Autodesk Inventor part; units mm, degrees
ref_plane "YZ Plane" through (0, 0, 0) normal (1, 0, 0) x (0, 1, 0)
ref_plane "XZ Plane" through (0, 0, 0) normal (0, 1, 0) x (-1, 0, 0)
ref_plane "XY Plane" through (0, 0, 0) normal (0, 0, 1) x (1, 0, 0)
sketch "スケッチ2" plane through (0, 0, 0) normal (0, 1, 0) x (-1, 0, 0)
  line L0 (0, 0) -> (20.1, 0)
  line L1 (20.1, 0) -> (20.1, -40)
  line L2 (20.1, -40) -> (0, -40)
  line L3 (0, -40) -> (0, 0)
  dimension "d0" = 20.1
  dimension "d1" = 40
extrude "押し出し1" add sketch "スケッチ2" along normal blind 27.5
ref_plane "作業平面1" through (0, 27.5, 0) normal (0, 1, 0) x (1, 0, 0)
sketch "スケッチ3" plane through (0, 27.5, 0) normal (0, 1, 0) x (1, 0, 0)
  line L0 (-20.1, 47.19) -> (0, 47.19)
  line L1 (0, 47.19) -> (0, -7.19)
  line L2 (0, -7.19) -> (-20.1, -7.19)
  line L3 (-20.1, -7.19) -> (-20.1, 47.19)
  line L4 (-20.1, 40) -> (-20.1, 0)
  line L5 (0, 40) -> (-20.1, 40)
  point P0 (0, 0)
  point P1 (-20.1, 20)
  point P2 (-20.1, 20)
  point P3 (-10.05, 47.19)
  point P4 (-10.05, 40)
  point P5 (-10.05, 40)
  point P6 (0, 40)
  point P7 (-20.1, 40)
  dimension "d5" = 20.1
  dimension "d6" = 54.38
  dimension "d7" = 0
  dimension "d8" = 0
extrude "押し出し2" add sketch "スケッチ3" along normal blind 3.1
ref_plane "作業平面2" through (0, 30.6, 0) normal (0, 1, 0) x (1, 0, 0)
sketch "スケッチ4" plane through (0, 30.6, 0) normal (0, 1, 0) x (1, 0, 0)
  line L0 (0, -7.19) -> (0, 0)
  line L1 (0, 0) -> (-20.1, 0)
  line L2 (-20.1, 0) -> (-20.1, 40)
  line L3 (-20.1, 40) -> (0, 40)
  line L4 (0, 40) -> (0, 0)
  circle A0 centre (-14.9, 45.43) radius 2
  circle A1 centre (-5.2, 45.43) radius 2
  line L5 (-15.85, 47.19) -> (-13.95, 47.19)
  line L6 (-6.15, 47.19) -> (-4.25, 47.19)
  line L7 (-13.95, 47.19) -> (-6.15, 47.19)
  line L8 (0, 47.19) -> (-20.1, 47.19)
  point P0 (-10.05, 47.19)
  dimension "d12" = 40
  dimension "d23" = 4
  dimension "d24" = 4
  dimension "d27" = 1.9
  dimension "d28" = 1.9
  dimension "d29" = 7.8
  dimension "d53" = 20.1
extrude "押し出し3" add sketch "スケッチ4" along normal blind 9.55 contours L1 L2 L3 L4
sketch "スケッチ7" plane through (0, 30.6, 0) normal (0, 1, 0) x (1, 0, 0)
  circle A0 centre (-14.9, 45.43) radius 2
  circle A1 centre (-5.2, 45.43) radius 2
  circle A2 centre (-14.9, -5.43) radius 2
  circle A3 centre (-5.2, -5.43) radius 2
  line L0 (-13.95, 47.19) -> (-15.85, 47.19)
  line L1 (-6.15, 47.19) -> (-4.25, 47.19)
  line L2 (-15.85, -7.19) -> (-13.95, -7.19)
  line L3 (-6.15, -7.19) -> (-4.25, -7.19)
  line L4 (-13.95, -7.19) -> (-6.15, -7.19)
  line L5 (-13.95, 47.19) -> (-6.15, 47.19)
  line L6 (0, 47.19) -> (-20.1, 47.19)
  line L7 (-20.1, -7.19) -> (0, -7.19)
  point P0 (0, 0)
  point P1 (-10.05, -7.19)
  point P2 (-10.05, 47.19)
  point P3 (-10.05, -7.19)
  dimension "d33" = 4
  dimension "d34" = 4
  dimension "d35" = 4
  dimension "d36" = 4
  dimension "d37" = 1.9
  dimension "d38" = 1.9
  dimension "d39" = 1.9
  dimension "d40" = 1.9
  dimension "d41" = 7.8
  dimension "d42" = 7.8
extrude "押し出し6" cut sketch "スケッチ7" against normal through all contours A0 L0 | L1 A1 | A2 L2 | A3 L3 | L3 A3 | L2 A2 picked at (-15.3262, 45.9006) picked at (-5.6145, 46.6348)
ref_plane "作業平面5" through (-20.1, 0, 0) normal (0, 0, 1) x (1, 0, 0)
sketch "スケッチ8" plane through (-20.1, 0, 0) normal (0, 0, 1) x (1, 0, 0)
  line L0 (6.05, 11.2) -> (14.05, 11.2)
  line L1 (14.05, 11.2) -> (14.05, 6.5)
  line L2 (14.05, 6.5) -> (6.05, 6.5)
  line L3 (6.05, 6.5) -> (6.05, 11.2)
  line L4 (0, 0) -> (0, 27.5)
  line L5 (20.1, 0) -> (20.1, 27.5)
  line L6 (0, 0) -> (20.1, 0)
  dimension "d46" = 8
  dimension "d47" = 4.7
  dimension "d48" = 6.05
  dimension "d49" = 6.05
  dimension "d50" = 6.5
extrude "押し出し7" cut sketch "スケッチ8" against normal blind 4.15
ref_plane "作業平面6" through (0, 40.15, 0) normal (0, 1, 0) x (1, 0, 0)
sketch "スケッチ10" plane through (0, 40.15, 0) normal (0, 1, 0) x (1, 0, 0)
  line L0 (-20.1, 0) -> (0, 0)
  circle A0 centre (-10.05, 9.9) radius 2.5
  point P0 (-10.05, 0)
  dimension "d57" = 9.9
  dimension "d59" = 5
extrude "押し出し8" add sketch "スケッチ10" along normal blind 5
ref_plane "作業平面7" through (-10.05, 45.15, -9.9) normal (0, 1, 0) x (1, 0, 0)
sketch "スケッチ11" plane through (-10.05, 45.15, -9.9) normal (0, 1, 0) x (1, 0, 0)
  line L0 (-10.05, -9.9) -> (10.05, -9.9)
  point P0 (0, 0)
  point P1 (0, -9.9)
  dimension "d63" = 9.9
Work out the finished part from the listing and answer in its coordinate system (mm). A direction names the side the tool comes from. Coordinates: 2 decimals unless noted, no trailing zeros. Loops run counter-clockwise (first coordinate to the right, second up) from the corner with the lowest first, then second, coordinate; pieces in that order, holes last. Notation, with made-up numbers: M 89.5,52 L 145.5,52 A7 cw 145.5,61 Z; hole C 39,55 d6. An arc over 180 degrees is marked long. Use CSV: the item, a comma, the result in double quotes. Start each with the question number.
(1) Find section C-C, the plane z = -9.9. Give the vertices of the cut face in (x, y), then the cut area to 3 significant figures.
(2) Find section D-D, the plane y = 19. Give the vertices of the cut face in (x, z).
(3) Find section B-B, the plane x = -5.2. Give the vertices of the cut face in (y, z).
(4) Given pin 1 Ø10 at (x, z) = (-7.5, -22) entering from +Y; pin 2 Ø6 at (x, y) = (-9.5, 16) entering from -Z; pin 3 Ø3.5 at (x, z) = (-7.5, -42.5) entering from -Y; pin 4 Ø3 at (x, z) = (-12, -7) entering from -Y, each flat-ended and moving along its own axis, determine where each tip first touches the part or whether it passes through.
(5) For a pull along X with two mould halves and no side action, classify faces 4 (the face through (0, 20, -20)), 5 (the face through (-5.27, 29.07, -43.43)), 6 (the face through (-18, 29, 7.19)) as +X half, -X half, draft (parallel to the pull), parting line (faces both ways), or undercut.
(6) Consider line 1 (X direction, y = 29, z = 5); line 2 (Z direction, x = -14.9, y = 29.65); line 3 (Z direction, x = -18.5, y = 10). Determine where each line is inside the solid, lowest interval first.
(7) For faces 1 (the face through (-12.548, 42.615, -9.79)), 2 (the face through (-10, 35, 0)), 3 (the face through (-10, 14, -40)), determine the directions among +Z, -Z, +X, -X, +Y, -Y from which every point of the face is accessible in a straight line to the end or side of a thin tool.
(8) Find section A-A, the plane z = 5.43. Give the vertices of the cut face in (x, y), then the cut area to 3 significant figures.
Recorded:
1,outline,"M -20.1,0 L 0,0 L 0,40.15 L -7.55,40.15 L -7.55,45.15 L -12.55,45.15 L -12.55,40.15 L -20.1,40.15 Z"
1,area,"832 mm^2"
2,outline,"M -20.1,-40 L 0,-40 L 0,0 L -20.1,0 Z"
3,outline,"M 0,-40 L 27.5,-40 L 27.5,-43.43 L 30.6,-43.43 L 30.6,-40 L 40.15,-40 L 40.15,0 L 30.6,0 L 30.6,3.43 L 27.5,3.43 L 27.5,0 L 0,0 Z"
4,pin 1,"stops at y = 40.15"
4,pin 2,"stops at z = -40"
4,pin 3,"stops at y = 27.5"
4,pin 4,"stops at y = 0"
5,face 4,"+X half"
5,face 5,"undercut"
5,face 6,"draft"
6,line 1,"x = -20.1 to -16.85, -12.95 to -7.15, -3.25 to 0"
6,line 2,"z = -43.43 to 3.43"
6,line 3,"z = -40 to 0"
7,face 1,"+Y"
7,face 2,"+Z, +X, -X, +Y"
7,face 3,"-Z, +X, -X, -Y"
8,outline,"M -20.1,27.5 L -16.9,27.5 L -16.9,30.6 L -20.1,30.6 Z; M -12.9,27.5 L -7.2,27.5 L -7.2,30.6 L -12.9,30.6 Z; M -3.2,27.5 L 0,27.5 L 0,30.6 L -3.2,30.6 Z"
8,area,"37.5 mm^2"
